For this review, take the finished solid that the model builds, in its own axes (mm). A direction names the side the tool comes from. Coordinates: 2 decimals unless noted, no trailing zeros. Loops run counter-clockwise (first coordinate to the right, second up) from the corner with the lowest first, then second, coordinate; pieces in that order, holes last. Notation, with made-up numbers: M -14.75,13 L 26.25,13 A10 cw 26.25,23 Z; hole C -1.75,-28.5 d5. An arc over 180 degrees is marked long. Write item = value, one per line.
from build123d import *

# Parameters (mm, degrees)
CROQUIS1_W              = 7.9
CROQUIS1_H              = 4.5
SALIENTE_EXTRUIR2_DEPTH = 6
CROQUIS4_W              = 6.9
CROQUIS4_H              = 3.5
CORTAR_EXTRUIR2_DEPTH   = 5
CROQUIS5_R              = 0.25
SALIENTE_EXTRUIR3_DEPTH = 3.4
CROQUIS6_W              = 2
CROQUIS6_H              = 0.5
CORTAR_EXTRUIR3_DEPTH   = 5
CROQUIS7_W              = 1
CROQUIS7_H              = 1
CORTAR_EXTRUIR5_DEPTH   = 8
CROQUIS8_W              = 1
CROQUIS8_H              = 4.000523864
CORTAR_EXTRUIR7_DEPTH   = 0.5
CHAFL_N3_SIZE           = 0.1


with BuildPart() as part:
    # Croquis1 → Saliente-Extruir2 (new body)
    with BuildSketch(Plane(origin=(0, 0, 0), x_dir=(1, 0, 0), z_dir=(0, 1, 0))):
        with Locations((0, -0.55)):
            Rectangle(CROQUIS1_W, CROQUIS1_H)
    extrude(amount=SALIENTE_EXTRUIR2_DEPTH)

    # Croquis4 → Cortar-Extruir2 (cut)
    with BuildSketch(Plane(origin=(0, 6, 0), x_dir=(1, 0, 0), z_dir=(0, 1, 0))):
        with Locations((0, -0.55)):
            Rectangle(CROQUIS4_W, CROQUIS4_H)
    extrude(amount=-CORTAR_EXTRUIR2_DEPTH, mode=Mode.SUBTRACT)

    # Croquis5 → Saliente-Extruir3 (add, symmetric)
    with BuildSketch(Plane(origin=(0, 0, 0), x_dir=(-1, 0, 0), z_dir=(0, -1, 0))):
        with Locations(Location((0, 0, 0), (0, 0, 90))):
            Circle(CROQUIS5_R)
        with Locations(Location((-2, 0, 0), (0, 0, 90))):
            Circle(CROQUIS5_R)
        with Locations(Location((2, 0, 0), (0, 0, 90))):
            Circle(CROQUIS5_R)
    extrude(amount=SALIENTE_EXTRUIR3_DEPTH, both=True)

    # Croquis6 → Cortar-Extruir3 (cut)
    with BuildSketch(Plane(origin=(0, 6, 0), x_dir=(1, 0, 0), z_dir=(0, 1, 0))):
        with Locations((0, 1.45)):
            Rectangle(CROQUIS6_W, CROQUIS6_H)
    extrude(amount=-CORTAR_EXTRUIR3_DEPTH, mode=Mode.SUBTRACT)

    # Croquis7 → Cortar-Extruir5 (cut)
    with BuildSketch(Plane(origin=(3.95, 0, 0), x_dir=(0, 0, -1), z_dir=(1, 0, 0))):
        with Locations((-0.55, 5.5)):
            Rectangle(CROQUIS7_W, CROQUIS7_H)
    extrude(amount=-CORTAR_EXTRUIR5_DEPTH, mode=Mode.SUBTRACT)

    # Croquis8 → Cortar-Extruir7 (cut)
    with BuildSketch(Plane(origin=(0, 0, -1.7), x_dir=(-1, 0, 0), z_dir=(0, 0, -1))):
        with Locations((-2.45, 2.000261932)):
            Rectangle(CROQUIS8_W, CROQUIS8_H)
        with Locations((2.45, 2.000261932)):
            Rectangle(CROQUIS8_W, CROQUIS8_H)
    extrude(amount=-CORTAR_EXTRUIR7_DEPTH, mode=Mode.SUBTRACT)

    # Chaflán3
    chafl_n3_edges = [part.edges().sort_by_distance(p)[0] for p in [
        (0, 3.4, 0.25),
        (0, -3.4, 0.25),
        (2, 3.4, 0.25),
        (2, -3.4, 0.25),
        (-2, 3.4, 0.25),
        (-2, -3.4, 0.25),
    ]]
    chamfer(chafl_n3_edges, length=CHAFL_N3_SIZE)


solid = part.part
Q1. Add section A-A (y = 1.5). Write out the cut boundary in (x, z).
Solved:
outline = M -3.95,-1.7 L -2.95,-1.7 L -2.95,-1.2 L -3.45,-1.2 L -3.45,2.3 L 3.45,2.3 L 3.45,-1.2 L 2.95,-1.2 L 2.95,-1.7 L 3.95,-1.7 L 3.95,2.8 L -3.95,2.8 Z; C -2,0 d0.5; M -1.95,-1.7 L -1,-1.7 L -1,-1.2 L -1.95,-1.2 Z; C 0,0 d0.5; M 1,-1.7 L 1.95,-1.7 L 1.95,-1.2 L 1,-1.2 Z; C 2,0 d0.5
Q2. Add section D-D (z = 0.45). Write out the cut boundary in (x, y), and give its area (3 significant figures).
Solved:
outline = M -3.95,0 L 3.95,0 L 3.95,5 L 3.45,5 L 3.45,1 L -3.45,1 L -3.45,5 L -3.95,5 Z
area = 11.9 mm²
Q3. For line 1 along Z through (x, y) = (-3, 2.5); line 2 along X through (y, z) = (2.5, 0.8); line 3 along Y through (x, z) = (0, 2.5), list the stretches that pass through material, from the lowest coordinate up.
Solved:
line_1 = -1.7 to -1.2, 2.3 to 2.8
line_2 = -3.95 to -3.45, 3.45 to 3.95
line_3 = 0 to 6
Q4. Add section C-C (y = 5.5). Write out the cut boundary in (x, z).
Solved:
outline = M -3.95,-1.7 L -1,-1.7 L -1,-1.2 L -3.45,-1.2 L -3.45,0.05 L -3.95,0.05 Z; M -3.95,1.05 L -3.45,1.05 L -3.45,2.3 L 3.45,2.3 L 3.45,1.05 L 3.95,1.05 L 3.95,2.8 L -3.95,2.8 Z; M 1,-1.7 L 3.95,-1.7 L 3.95,0.05 L 3.45,0.05 L 3.45,-1.2 L 1,-1.2 Z
Q5. Add section B-B (x = 0). Write out the cut boundary in (y, z).
Solved:
outline = M -3.4,-0.15 L -3.3,-0.25 L 0,-0.25 L 0,-1.7 L 1,-1.7 L 1,-0.25 L 3.3,-0.25 L 3.4,-0.15 L 3.4,0.15 L 3.3,0.25 L 1,0.25 L 1,2.3 L 6,2.3 L 6,2.8 L 0,2.8 L 0,0.25 L -3.3,0.25 L -3.4,0.15 Z
Q6. Draft analysis for pull direction X (two halves, no side actions). For faces 4 (the face through (2.8, 6, -1.4)), 5 (the face through (2.5, 0.5, -1.2)), 6 (the face through (-3.95, 3, 1)), state which applies: +X half, -X half, draft (parallel to the pull), parting line (faces both ways), or undercut.
Solved:
face_4 = draft
face_5 = undercut
face_6 = -X half
Q7. Machinability: for faces 1 (the face through (-3.45, 4, 1)), 2 (the face through (-2.8, 6, -1.4)), 3 (the face through (-2.4, 0.5, -1.2)), which of the approach directions +Z, -Z, +X, -X, +Y, -Y give a long, thin tool a straight path to every point of the face, cutting with its end or side? Answer none if there is none.
Solved:
face_1 = +Y
face_2 = +Z, -Z, +X, -X, +Y
face_3 = -Z, -Y
